from build123d import *

# Parameters (mm, degrees)
SKETCH1_W           = 8.8
SKETCH1_H           = 31.2
SKETCH1_W_2         = 6.8
SKETCH1_H_2         = 29.2
BOSS_EXTRUDE1_DEPTH = 5
SKETCH2_W           = 8.8
SKETCH2_H           = 31.2
BOSS_EXTRUDE2_DEPTH = 1
CUT_EXTRUDE1_REACH  = 34.023
SKETCH3_W           = 29.2
SKETCH3_H           = 2


with BuildPart() as part:
    # Sketch1 → Boss-Extrude1 (new body)
    with BuildSketch(Plane(origin=(0, 0, 0), x_dir=(1, 0, 0), z_dir=(0, 1, 0))):
        with Locations((3.4, 14.6)):
            Rectangle(SKETCH1_W, SKETCH1_H)
        with Locations((3.4, 14.6)):
            Rectangle(SKETCH1_W_2, SKETCH1_H_2, mode=Mode.SUBTRACT)
    extrude(amount=BOSS_EXTRUDE1_DEPTH)

    # Sketch2 → Boss-Extrude2 (add)
    with BuildSketch(Plane(origin=(0, 5, 0), x_dir=(1, 0, 0), z_dir=(0, 1, 0))):
        with Locations((3.4, 14.6)):
            Rectangle(SKETCH2_W, SKETCH2_H)
    extrude(amount=BOSS_EXTRUDE2_DEPTH)

    # Sketch3 → Cut-Extrude1 (cut, up to next)
    with BuildSketch(Plane.ZY.offset(1), mode=Mode.PRIVATE) as cut_extrude1_sk1:
        with Locations((-14.6, 1)):
            Rectangle(SKETCH3_W, SKETCH3_H)
    cut_extrude1_tool1 = extrude(cut_extrude1_sk1.sketch, amount=-CUT_EXTRUDE1_REACH, mode=Mode.PRIVATE) & part.part
    add(cut_extrude1_tool1.solids().sort_by_distance((-1, 1, -14.6))[0], mode=Mode.SUBTRACT)


solid = part.part
Read the model definition and answer for the solid it produces. Units are mm, in the model's axes. A direction names the side the tool comes from. Round coordinates to 2 decimals unless told otherwise and drop trailing zeros. Write each loop counter-clockwise with the first axis right and the second up, starting at its lowest first coordinate (ties: lowest second). Pieces come first, ordered by that corner, then holes. Notation, with made-up numbers: (9.5, 56) - (45.5, 56) arc R23 cw to (45.5, 95) - close; hole circle Ø11 at (68, 87). An arc over 180 degrees is marked (long way). One line per question, with ' | ' between items. Start each with the question number.
1. Section B-B (x = -0.5) is taken. Determine the outline of the cut face in (y, z).
2. Section C-C (y = 1.1) is taken. Determine the outline of the cut face in (x, z), and give its area (3 significant figures).
3. For faces 1 (the face through (3, 3, 1)), 2 (the face through (6.8, 2, -14)), determine the directions among +Z, -Z, +X, -X, +Y, -Y from which every point of the face is accessible in a straight line to the end or side of a thin tool.
4. For a pull along Z with two mould halves and no side action, classify faces 3 (the face through (-0.5, 2, -14.8)), 4 (the face through (3, 3, -30.2)), 5 (the face through (3, 6, -15)) as +Z half, -Z half, draft (parallel to the pull), parting line (faces both ways), or undercut.
5. This flat-tipped pin is pushed along its axis until it touches: pin 1 (0.5 mm diameter, centred on x = -0.5, z = -13.5, fed in from -Y). Where does it stop, or does it pass through?
6. Find the intervals of material crossed by probe 1 along Z at (x, y) = (4, 1.6); probe 2 along X at (y, z) = (3.1, -23); probe 3 along X at (y, z) = (1.55, -20), in increasing order. Write a range as [from, to].
7. Section A-A (y = 3.2) is taken. Determine the outline of the cut face in (x, z).
Filled in:
1) outline: (0, -30.2) - (6, -30.2) - (6, 1) - (0, 1) - (0, 0) - (2, 0) - (2, -29.2) - (0, -29.2) - close
2) outline: (-1, -30.2) - (7.8, -30.2) - (7.8, 1) - (-1, 1) - (-1, 0) - (6.8, 0) - (6.8, -29.2) - (-1, -29.2) - close | area: 46.8 mm²
3) face 1: +Z, +X, -X, +Y, -Y | face 2: -Y
4) face 3: undercut | face 4: -Z half | face 5: draft
5) pin 1: y = 2
6) probe 1: [-30.2, -29.2], [0, 1] | probe 2: [-1, 0], [6.8, 7.8] | probe 3: [6.8, 7.8]
7) outline: (-1, -30.2) - (7.8, -30.2) - (7.8, 1) - (-1, 1) - close; hole (0, -29.2) - (6.8, -29.2) - (6.8, 0) - (0, 0) - close
